Check sheet for the modelled part. Datum: model origin and axes. Units: mm. Round coordinates to 2 decimals unless told otherwise and drop trailing zeros. Order: outer loops, then holes, each group sorted by start corner. A loop starts at its lowest first (then second) coordinate and runs counter-clockwise, first axis right, second up. Notation, with made-up numbers: (41.25, -31) -> (99.25, -31) arc R24 ccw to (99.25, -13) -> close; hole circle Ø7 at (85, -38). An arc over 180 degrees is marked (long way). Use CSV: the item, a comma, the result in double quotes.
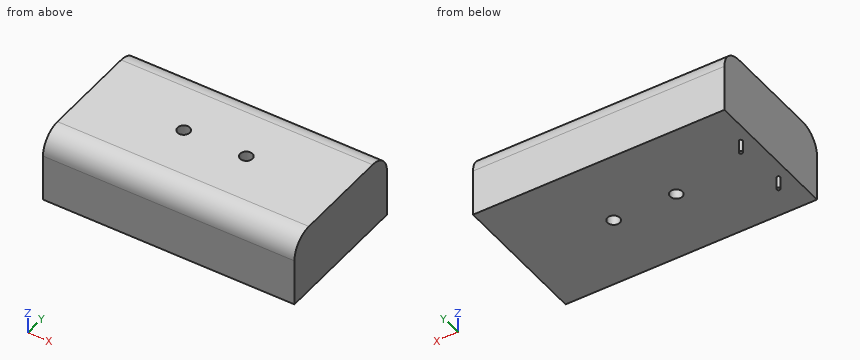
Autodesk Inventor part; units mm, degrees
ref_plane "YZ Plane" through (0, 0, 0) normal (1, 0, 0) x (0, 1, 0)
ref_plane "XZ Plane" through (0, 0, 0) normal (0, 1, 0) x (-1, 0, 0)
ref_plane "XY Plane" through (0, 0, 0) normal (0, 0, 1) x (1, 0, 0)
sketch "スケッチ1" plane through (0, 0, 0) normal (0, 0, 1) x (1, 0, 0)
  line L0 (-28.5, 16) -> (28.5, 16)
  line L1 (28.5, 16) -> (28.5, -16)
  line L2 (28.5, -16) -> (-28.5, -16)
  line L3 (-28.5, -16) -> (-28.5, 16)
  point P0 (0, 0)
  point P1 (-28.5, 0)
  point P2 (0, 16)
  dimension "d0" = 57
  dimension "d1" = 32
extrude "押し出し1" add sketch "スケッチ1" along normal blind 15.7
fillet "フィレット1" radius 5 2 edges at (0, 16, 15.7) (0, -16, 15.7)
sketch "スケッチ2" plane through (0, 0, 0) normal (0, 0, -1) x (-1, 0, 0)
  line L0 (26, 20.4284) -> (26, -20.6337) construction
  line L1 (0, 0) -> (36.4083, 0) construction
  line L2 (28.5, 16) -> (28.5, -16) construction
  circle A0 centre (26, 6.5) radius 0.4
  circle A1 centre (26, -6.5) radius 0.4
  dimension "d5" = 2.5
  dimension "d6" = 0.8
  dimension "d7" = 13
extrude "押し出し2" add sketch "スケッチ2" along normal blind 2.8
sketch "スケッチ3" plane through (0, 0, 0) normal (0, 0, -1) x (-1, 0, 0)
  circle A0 centre (-7.1, 0) radius 1.4
  circle A1 centre (7.1, 0) radius 1.4
  point P0 (0, 0)
  dimension "d10" = 2.8
  dimension "d11" = 7.1
  dimension "d12" = 7.1
extrude "押し出し3" cut sketch "スケッチ3" against normal through all
properties part number "BH321-1P24"
Q1. Scan lines: L1, parallel to Y at x = 7.1, z = 7.5; L2, parallel to Z at x = 3, y = 7; L3, parallel to Y at x = 7.1, z = 12.5. Record each from-to range of solid material in increasing order.
Result sheet:
L1,"y = -16 to -1.4, 1.4 to 16"
L2,"z = 0 to 15.7"
L3,"y = -15.66 to -1.4, 1.4 to 15.66"
Q2. Go/stop test with flat-tipped pins: pin 1 (10 mm diameter, centred on x = -2, y = 12, fed in from -Z); pin 2 (2.5 mm diameter, centred on x = 7.1, y = 0, fed in from +Z). Record where each tip stops, or that it passes through.
Result sheet:
pin 1,"stops at z = 0"
pin 2,"passes through"
Q3. Sectioned sample at D-D, the plane x = 2.5. Enter the section's corners in (y, z).
Result sheet:
outline,"(-16, 0) -> (16, 0) -> (16, 10.7) arc R5 ccw to (11, 15.7) -> (-11, 15.7) arc R5 ccw to (-16, 10.7) -> close"
Q4. Sectioned sample at A-A, the plane x = -7.1. Enter the section's corners in (y, z), then the cut area to 3 significant figures.
Result sheet:
outline,"(-16, 0) -> (-1.4, 0) -> (-1.4, 15.7) -> (-11, 15.7) arc R5 ccw to (-16, 10.7) -> close; (1.4, 0) -> (16, 0) -> (16, 10.7) arc R5 ccw to (11, 15.7) -> (1.4, 15.7) -> close"
area,"448 mm^2"
Q5. Sectioned sample at C-C, the plane z = -1.25. Enter the section's corners in (x, y), then the cut area to 3 significant figures.
Result sheet:
outline,"circle Ø0.8 at (-26, -6.5); circle Ø0.8 at (-26, 6.5)"
area,"1.01 mm^2"
Q6. Sectioned sample at B-B, the plane y = 0. Enter the section's corners in (x, z), then the cut area to 3 significant figures.
Result sheet:
outline,"(-28.5, 0) -> (-8.5, 0) -> (-8.5, 15.7) -> (-28.5, 15.7) -> close; (-5.7, 0) -> (5.7, 0) -> (5.7, 15.7) -> (-5.7, 15.7) -> close; (8.5, 0) -> (28.5, 0) -> (28.5, 15.7) -> (8.5, 15.7) -> close"
area,"807 mm^2"
